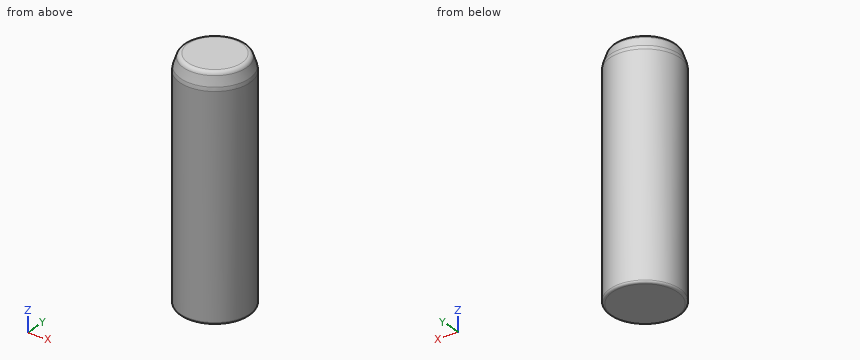
```python
from build123d import *

# Parameters (mm, degrees)
F0_R     = 14.95
F1_DEPTH = 100
F2_SIZE2 = 6
F2_SIZE  = 2
F3_R     = 1
F4_R     = 2
F5_R     = 5


with BuildPart() as f1:
    # F0 (on Top) → F1 (new body)
    with BuildSketch(Plane.XY):
        with Locations((0, 1.4814995229)):
            Circle(F0_R)
    extrude(amount=F1_DEPTH)

    # F2
    f2_edges = [f1.edges().sort_by_distance(p)[0] for p in [
        (-14.95, 1.4815, 100),
    ]]
    f2_side = f1.faces().sort_by_distance((0, 1.4815, 100))[0]
    chamfer(f2_edges, length=F2_SIZE, length2=F2_SIZE2, reference=f2_side)

    # F3
    f3_edges = [f1.edges().sort_by_distance(p)[0] for p in [
        (-14.95, 1.4815, 0),
    ]]
    fillet(f3_edges, radius=F3_R)

    # F4
    f4_edges = [f1.edges().sort_by_distance(p)[0] for p in [
        (-12.95, 1.4815, 100),
    ]]
    fillet(f4_edges, radius=F4_R)

    # F5
    f5_edges = [f1.edges().sort_by_distance(p)[0] for p in [
        (-14.95, 1.4815, 94),
    ]]
    fillet(f5_edges, radius=F5_R)


solid = f1.part
```
For this review, take the finished solid that the model builds, in its own axes (mm). Coordinates: 2 decimals unless noted, no trailing zeros. Write each loop counter-clockwise with the first axis right and the second up, starting at its lowest first coordinate (ties: lowest second). Pieces come first, ordered by that corner, then holes. Notation, with made-up numbers: (-37, -12.5) - (7, -12.5) arc R21 cw to (7, -0.5) - close; hole circle Ø9 at (70, 83.5). An arc over 180 degrees is marked (long way). Answer in a Markdown table with one row per item. Add a question column.
Q1. For probe 1 along X at (y, z) = (1.75, 91.5); probe 2 along X at (y, z) = (9, 72.5); probe 3 along Y at (x, z) = (7.25, 17.5), list the stretches that pass through material, from the lowest coordinate up.
Q2. We need section A-A, the plane z = 45.5. State the section outline as (x, y) points, and give its area (3 significant figures).
Q3. For P1, Ø5, axis at x = -4.5, z = 87.5, coming from the -Y side; P2, Ø1.5, axis at y = 10, z = 32.5, coming from the +X side; P3, Ø1.5, axis at x = 10.5, z = 33, coming from the +Y side, all flat-tipped, find the tip position at first contact; note any pin that passes through.
Answer list:
| question | item | result |
|---|---|---|
| 1 | probe 1 | x = -14.95 to 14.95 |
| 1 | probe 2 | x = -12.92 to 12.92 |
| 1 | probe 3 | y = -11.59 to 14.56 |
| 2 | outline | circle Ø29.9 at (0, 1.48) |
| 2 | area | 702 mm2 |
| 3 | P1 | stops at y = -13.33 |
| 3 | P2 | stops at x = 12.77 |
| 3 | P3 | stops at y = 12.81 |
